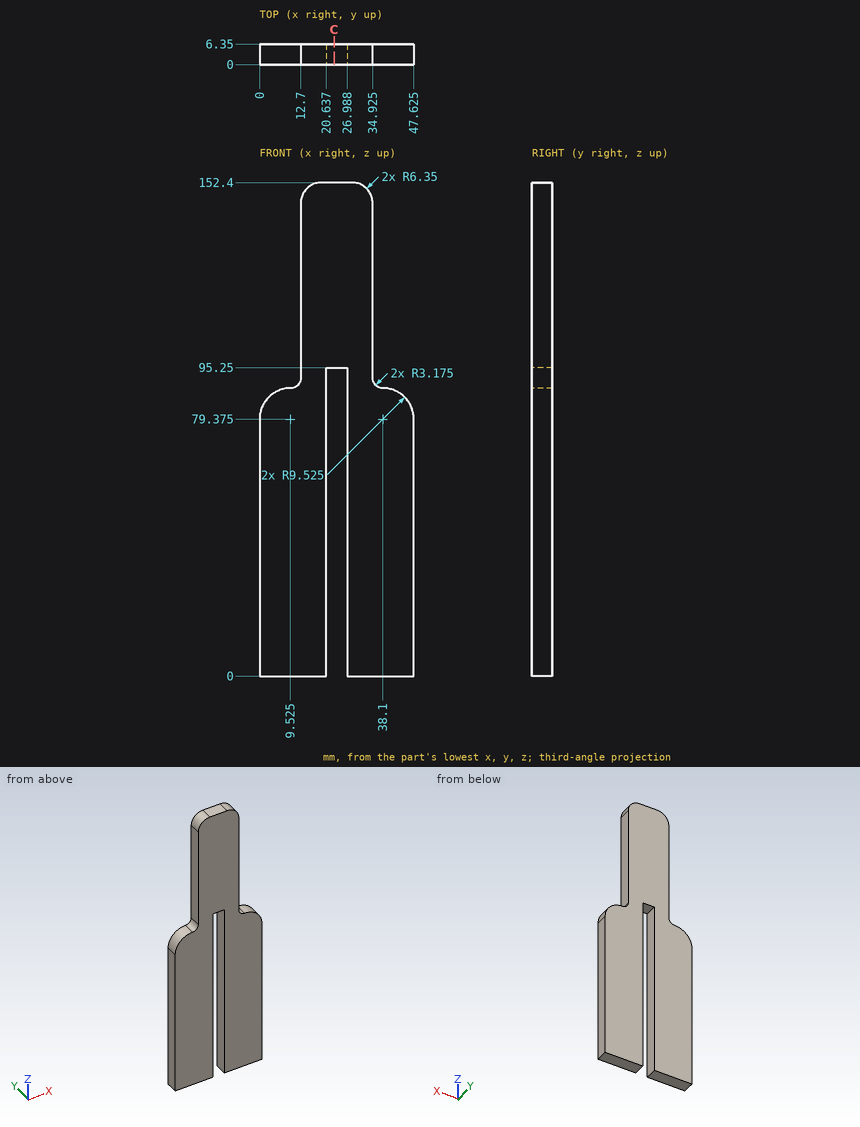
Check sheet for the drawn part. Datum: minimum x, y, z corner. Units: mm. Give positions to 0.01 mm unless a question says otherwise; leave off trailing zeros. Order: outer loops, then holes, each group sorted by start corner. A loop starts at its lowest first (then second) coordinate and runs counter-clockwise, first axis right, second up.
1. Sectioned sample at C-C (x = 23). Record the boundary of the cut face in (y, z).
Completed:
outline: (0, 95.25) - (6.35, 95.25) - (6.35, 152.4) - (0, 152.4) - close
2. Depth check by flat-ended pin: pin 1 (6 mm diameter, centred on x = 40, z = 82.5, fed in from -Y); pin 2 (1.9 mm diameter, centred on x = 24, y = 3.5, fed in from -Z); pin 3 (3 mm diameter, centred on y = 3, z = 114, fed in from +X) (1 decimal). Enter the tip coordinate at first touch or a pass-through.
Completed:
pin 1: stops at y = 0
pin 2: stops at z = 95.25
pin 3: stops at x = 34.9
3. Scan lines: line 1 (X direction, y = 5, z = 62) (1 decimal); line 2 (X direction, y = 4.75, z = 101) (1 decimal); line 3 (Z direction, x = 26, y = 2.5). Record each from-to range of solid material in increasing order.
Completed:
line 1: x = 0 to 20.6, 27 to 47.6
line 2: x = 12.7 to 34.9
line 3: z = 95.25 to 152.4
